from build123d import *

# Parameters (mm, degrees)
SKETCH1_W           = 203.2
SKETCH1_H           = 17.78
SKETCH1_R           = 3.96875
BOSS_EXTRUDE1_DEPTH = 33.02
SKETCH2_R           = 3.175
CUT_EXTRUDE1_DEPTH  = 17.78
SKETCH3_R           = 4.7625
CUT_EXTRUDE2_DEPTH  = 4.7752
CUT_EXTRUDE3_DEPTH  = 17.78
CUT_EXTRUDE4_DEPTH  = 17.78
FILLET1_R           = 2.54


with BuildPart() as part:
    # Sketch1 → Boss-Extrude1 (new body)
    with BuildSketch(Plane(origin=(0, 0, 0), x_dir=(1, 0, 0), z_dir=(0, 1, 0))):
        with Locations((0, 8.89)):
            Rectangle(SKETCH1_W, SKETCH1_H)
        with Locations(Location((76.2, 8.89, 0), (0, 0, 270))):
            Circle(SKETCH1_R, mode=Mode.SUBTRACT)
        with Locations(Location((25.4, 8.89, 0), (0, 0, 270))):
            Circle(SKETCH1_R, mode=Mode.SUBTRACT)
        with Locations(Location((-25.4, 8.89, 0), (0, 0, 270))):
            Circle(SKETCH1_R, mode=Mode.SUBTRACT)
        with Locations(Location((-76.2, 8.89, 0), (0, 0, 270))):
            Circle(SKETCH1_R, mode=Mode.SUBTRACT)
    extrude(amount=-BOSS_EXTRUDE1_DEPTH)

    # Sketch2 → Cut-Extrude1 (cut)
    with BuildSketch(Plane.XY):
        with Locations((88.9, -16.51)):
            Circle(SKETCH2_R)
        with Locations((0, -16.51)):
            Circle(SKETCH2_R)
        with Locations((-88.9, -16.51)):
            Circle(SKETCH2_R)
    extrude(amount=-CUT_EXTRUDE1_DEPTH, mode=Mode.SUBTRACT)

    # Sketch3 → Cut-Extrude2 (cut)
    with BuildSketch(Plane.XY):
        with Locations((88.9, -16.51)):
            Circle(SKETCH3_R)
        with Locations((0, -16.51)):
            Circle(SKETCH3_R)
        with Locations((-88.9, -16.51)):
            Circle(SKETCH3_R)
    extrude(amount=-CUT_EXTRUDE2_DEPTH, mode=Mode.SUBTRACT)

    # Sketch4 → Cut-Extrude3 (cut)
    with BuildSketch(Plane.XY):
        with BuildLine():
            Line((-36.195, -29.21), (-65.405, -29.21))
            ThreePointArc((-65.405, -29.21), (-66.303025612, -28.838025612), (-66.675, -27.94))
            Line((-66.675, -27.94), (-66.675, -5.08))
            ThreePointArc((-66.675, -5.08), (-66.303025612, -4.181974388), (-65.405, -3.81))
            Line((-65.405, -3.81), (-36.195, -3.81))
            ThreePointArc((-36.195, -3.81), (-35.296974388, -4.181974388), (-34.925, -5.08))
            Line((-34.925, -5.08), (-34.925, -27.94))
            ThreePointArc((-34.925, -27.94), (-35.296974388, -28.838025612), (-36.195, -29.21))
        make_face()
        with BuildLine():
            Line((-8.636, -27.305), (-16.764, -27.305))
            ThreePointArc((-16.764, -27.305), (-17.662025612, -26.933025612), (-18.034, -26.035))
            Line((-18.034, -26.035), (-18.034, -6.985))
            ThreePointArc((-18.034, -6.985), (-17.662025612, -6.086974388), (-16.764, -5.715))
            Line((-16.764, -5.715), (-8.636, -5.715))
            ThreePointArc((-8.636, -5.715), (-7.737974388, -6.086974388), (-7.366, -6.985))
            Line((-7.366, -6.985), (-7.366, -10.471153339))
            ThreePointArc((-7.366, -10.471153339), (-9.525, -16.51), (-7.366, -22.548846661))
            Line((-7.366, -22.548846661), (-7.366, -26.035))
            ThreePointArc((-7.366, -26.035), (-7.737974388, -26.933025612), (-8.636, -27.305))
        make_face()
        with BuildLine():
            Line((36.195, -3.81), (65.405, -3.81))
            ThreePointArc((65.405, -3.81), (66.303025612, -4.181974388), (66.675, -5.08))
            Line((66.675, -5.08), (66.675, -27.94))
            ThreePointArc((66.675, -27.94), (66.303025612, -28.838025612), (65.405, -29.21))
            Line((65.405, -29.21), (36.195, -29.21))
            ThreePointArc((36.195, -29.21), (35.296974388, -28.838025612), (34.925, -27.94))
            Line((34.925, -27.94), (34.925, -5.08))
            ThreePointArc((34.925, -5.08), (35.296974388, -4.181974388), (36.195, -3.81))
        make_face()
        with BuildLine():
            Line((7.366, -26.035), (7.366, -22.548846661))
            ThreePointArc((7.366, -22.548846661), (9.525, -16.51), (7.366, -10.471153339))
            Line((7.366, -10.471153339), (7.366, -6.985))
            ThreePointArc((7.366, -6.985), (7.737974388, -6.086974388), (8.636, -5.715))
            Line((8.636, -5.715), (16.764, -5.715))
            ThreePointArc((16.764, -5.715), (17.662025612, -6.086974388), (18.034, -6.985))
            Line((18.034, -6.985), (18.034, -26.035))
            ThreePointArc((18.034, -26.035), (17.662025612, -26.933025612), (16.764, -27.305))
            Line((16.764, -27.305), (8.636, -27.305))
            ThreePointArc((8.636, -27.305), (7.737974388, -26.933025612), (7.366, -26.035))
        make_face()
    extrude(amount=-CUT_EXTRUDE3_DEPTH, mode=Mode.SUBTRACT)

    # Sketch5 → Cut-Extrude4 (cut)
    with BuildSketch(Plane.XY):
        with BuildLine():
            Line((88.9, -27.869225326), (88.9, -33.02))
            Line((88.9, -33.02), (101.6, -33.02))
            Line((101.6, -33.02), (101.6, 0))
            Line((101.6, 0), (88.9, 0))
            Line((88.9, 0), (88.9, -5.150774674))
            ThreePointArc((88.9, -5.150774674), (89.22339789, -5.997441341), (90.028888889, -6.412910822))
            ThreePointArc((90.028888889, -6.412910822), (99.06, -16.51), (90.028888889, -26.607089178))
            ThreePointArc((90.028888889, -26.607089178), (89.22339789, -27.022558659), (88.9, -27.869225326))
        make_face()
        with BuildLine():
            Line((-88.9, -5.150774674), (-88.9, 0))
            Line((-88.9, 0), (-101.6, 0))
            Line((-101.6, 0), (-101.6, -33.02))
            Line((-101.6, -33.02), (-88.9, -33.02))
            Line((-88.9, -33.02), (-88.9, -27.869225326))
            ThreePointArc((-88.9, -27.869225326), (-89.22339789, -27.022558659), (-90.028888889, -26.607089178))
            ThreePointArc((-90.028888889, -26.607089178), (-99.06, -16.51), (-90.028888889, -6.412910822))
            ThreePointArc((-90.028888889, -6.412910822), (-89.22339789, -5.997441341), (-88.9, -5.150774674))
        make_face()
    extrude(amount=-CUT_EXTRUDE4_DEPTH, mode=Mode.SUBTRACT)

    # Fillet1
    fillet1_edges = [part.edges().sort_by_distance(p)[0] for p in [
        (88.9, 0, -8.89),
        (88.9, -33.02, -8.89),
        (-88.9, 0, -8.89),
        (-88.9, -33.02, -8.89),
    ]]
    fillet(fillet1_edges, radius=FILLET1_R)


solid = part.part
The listing builds one solid part. Answer for the finished solid, in the listing's coordinates (mm). A direction names the side the tool comes from. Give positions to 0.01 mm unless a question says otherwise; leave off trailing zeros. Order: outer loops, then holes, each group sorted by start corner. A loop starts at its lowest first (then second) coordinate and runs counter-clockwise, first axis right, second up. Notation, with made-up numbers: (-34.75, -23) - (-7.75, -23) arc R33 cw to (-7.75, 8) - close; hole circle Ø4 at (70, 21.25). An arc over 180 degrees is marked (long way). Answer as CSV lines item,"result".
Q1. Each of these flat-tipped pins is pushed along its axis until it touches: pin 1 Ø9 at (x, z) = (-13.5, -10.5) entering from +Y; pin 2 Ø1 at (y, z) = (-9, -7) entering from -X; pin 3 Ø0.8 at (y, z) = (-29.5, -10.5) entering from -X; pin 4 Ø3 at (y, z) = (-24, -10) entering from -X. Where does it stop, or does it pass through?
Answer key:
pin 1,"stops at y = 0"
pin 2,"stops at x = -96.25"
pin 3,"stops at x = -88.9"
pin 4,"stops at x = -97.11"
Q2. Which of the six approach directions +Z, -Z, +X, -X, +Y, -Y give full straight-line access (tool end or side, diameter ignored) to faces 1 (the face through (29.335, -16.279, -9.407)), 2 (the face through (51, -29.21, -9)), 3 (the face through (-88, -20, -4.775))?
Answer key:
face 1,"+Y, -Y"
face 2,"+Z, -Z"
face 3,"+Z"
Q3. A cutting plane is placed at A-A, the plane y = -16.51. Count the separate pieces of the cut face and the enclosed holes in it, and give its area (3 significant figures).
Answer key:
separate pieces,"8"
enclosed holes,"4"
area,"1,510 mm^2"
Q4. A cutting plane is placed at B-B, the plane x = 25.4. Determine the outline of the cut face in (y, z).
Answer key:
outline,"(-33.02, -17.78) - (0, -17.78) - (0, -12.86) - (-33.02, -12.86) - close; (-33.02, -4.92) - (0, -4.92) - (0, 0) - (-33.02, 0) - close"
Q5. Straight lines are drawn through the part: L1, parallel to Y at x = -47, z = -6.5; L2, parallel to Y at x = 0, z = -2.15; L3, parallel to X at y = -20, z = -16 (3 decimals). For each, find the intervals that lie inside material, in ascending order.
Answer key:
L1,"y = -33.02 to -29.21, -3.81 to 0"
L2,"y = -33.02 to -21.27, -11.75 to 0"
L3,"x = -98.442 to -66.675, -34.925 to -18.034, -8.863 to 8.863, 18.034 to 34.925, 66.675 to 98.442"
Q6. Determine the mould class of faces 4 (the face through (-1, -24, 0)), 5 (the face through (-1, -33.02, -9)), 6 (the face through (66.675, -16, -9)), 7 (the face through (99.058, -16.302, -8.766)) for opening direction Y: pulls with the +Y half, pulls with the -Y half, needs draft (parallel to the pull), parting line crosses it, or undercut.
Answer key:
face 4,"needs draft"
face 5,"pulls with the -Y half"
face 6,"undercut"
face 7,"parting line crosses it"
